from build123d import *

# Parameters (mm, degrees)
SM_BASE_FLANGE_1_DEPTH = 1.5
OTHER_START            = -10
OTHER_1_DEPTH          = 20
OTHER_1_2_DEPTH        = 20
FILLET_1_R             = 1
SKETCH_7_R             = 1.5
CUT_EXTRUDE_1_DEPTH    = 10
SKETCH_8_R             = 1.5
CUT_EXTRUDE_2_DEPTH    = 10


# Read off the part's stored shape, not the designer's step: 绘制的折弯1
# Sheet-metal steps are written as plain solids
with BuildPart() as part:
    # Sketch 1 → 基体-法兰1 (new body)
    with BuildSketch(Plane.XY):
        Polygon((10, 10), (20, 10), (20, 30), (-20, 30), (-20, 10), (-10, 10), (-10, -10), (10, -10), align=None)
    extrude(amount=-SM_BASE_FLANGE_1_DEPTH)

    # Other 1 outline → Other 1 (cut)
    with BuildSketch(Plane.YZ.offset(OTHER_START)):
        with BuildLine():
            ThreePointArc((10, -1.5), (8.630693606, -1.091650066), (7.708712152, 0))
            Line((7.708712152, 0), (-10, 0))
            Line((-10, 0), (-10, -1.5))
            Line((-10, -1.5), (10, -1.5))
        make_face()
    extrude(amount=OTHER_1_DEPTH, mode=Mode.SUBTRACT)

    # Other 1 2 outline → Other 1 2 (add)
    with BuildSketch(Plane.YZ.offset(OTHER_START)):
        with BuildLine():
            Line((9, 18.251106428), (7.5, 18.251106428))
            Line((7.5, 18.251106428), (7.5, 1))
            ThreePointArc((7.5, 1), (7.552734218, 0.489225891), (7.708712152, 0))
            Line((7.708712152, 0), (10, 0))
            ThreePointArc((10, 0), (9.292893219, 0.292893219), (9, 1))
            Line((9, 1), (9, 18.251106428))
        make_face()
    extrude(amount=OTHER_1_2_DEPTH)

    # 圆角1
    fillet_1_edges = [part.edges().sort_by_distance(p)[0] for p in [
        (10, 8.25, 18.251106428),
        (-10, 8.25, 18.251106428),
        (20, 30, -0.75),
        (-20, 30, -0.75),
        (-20, 10, -0.75),
        (20, 10, -0.75),
    ]]
    fillet(fillet_1_edges, radius=FILLET_1_R)

    # 草图7 → 切除-拉伸1 (cut)
    with BuildSketch(Plane(origin=(0, 0, -1.5), x_dir=(-1, 0, 0), z_dir=(0, 0, -1))):
        with Locations((-13, 25)):
            Circle(SKETCH_7_R)
        with Locations((13, 25)):
            Circle(SKETCH_7_R)
        with Locations((-13, 15)):
            Circle(SKETCH_7_R)
        with Locations((13, 15)):
            Circle(SKETCH_7_R)
    extrude(amount=-CUT_EXTRUDE_1_DEPTH, mode=Mode.SUBTRACT)

    # 草图8 → 切除-拉伸2 (cut)
    with BuildSketch(Plane.XZ.offset(-7.5)):
        with Locations(Location((-5, 13.251106428, 0), (0, 0, 270))):
            Circle(SKETCH_8_R)
        with Locations(Location((5, 13.251106428, 0), (0, 0, 270))):
            Circle(SKETCH_8_R)
        with Locations(Location((-5, 6.251106428, 0), (0, 0, 270))):
            Circle(SKETCH_8_R)
        with Locations(Location((5, 6.251106428, 0), (0, 0, 270))):
            Circle(SKETCH_8_R)
    extrude(amount=-CUT_EXTRUDE_2_DEPTH, mode=Mode.SUBTRACT)


solid = part.part
The listing builds one solid part. Answer for the finished solid, in the listing's coordinates (mm). A direction names the side the tool comes from. Give positions to 0.01 mm unless a question says otherwise; leave off trailing zeros. Write each loop counter-clockwise with the first axis right and the second up, starting at its lowest first coordinate (ties: lowest second). Pieces come first, ordered by that corner, then holes. Notation, with made-up numbers: (83, -28.5) -> (104, -28.5) arc R33 cw to (104, 9.5) -> close; hole circle Ø9 at (82.25, 58.5). An arc over 180 degrees is marked (long way). One line per question, with ' | ' between items. Start each with the question number.
1. Find the intervals of material crossed by probe 1 along Y at (x, z) = (13, -1.05); probe 2 along Z at (x, y) = (7.5, 26); probe 3 along Y at (x, z) = (-5.5, 8.5), in increasing order.
2. Section D-D (x = -7.5) is taken. Determine the outline of the cut face in (y, z).
3. Section B-B (y = 25) is taken. Determine the outline of the cut face in (x, z).
4. Given pin 1 Ø2 at (y, z) = (8, 12) entering from -X; pin 2 Ø0.8 at (x, z) = (-13.5, -1) entering from -Y; pin 3 Ø3 at (x, y) = (9, 18.5) entering from +Z, each flat-ended and moving along its own axis, determine where each tip first touches the part or whether it passes through.
5. Section A-A (x = 5) is taken. Determine the outline of the cut face in (y, z), plus the area to 3 significant figures.
6. Section C-C (z = 6) is taken. Determine the outline of the cut face in (x, y).
7. For a pull along X with two mould halves and no side action, classify faces 4 (the cylindrical face through (5.45, 8.24, 4.82)), 5 (the flat face through (0, 20, -1.5)), 6 (the flat face through (20, 20, -1)) as pulls with the +X half, pulls with the -X half, needs draft (parallel to the pull), parting line crosses it, or undercut.
8. For faces 1 (the flat face through (0, 20, 0)), 2 (the flat face through (-15, 10, -1)), 3 (the flat face through (0, 7.5, 10)), determine the directions among +Z, -Z, +X, -X, +Y, -Y from which every point of the face is accessible in a straight line to the end or side of a thin tool.
Response values:
1) probe 1: 10 to 13.5, 16.5 to 23.5, 26.5 to 30 | probe 2: -1.5 to 0 | probe 3: 7.5 to 9
2) outline: (7.5, 1) arc R2.5 ccw to (10, -1.5) -> (30, -1.5) -> (30, 0) -> (10, 0) arc R1 cw to (9, 1) -> (9, 18.25) -> (7.5, 18.25) -> close
3) outline: (-20, -1.5) -> (-14.5, -1.5) -> (-14.5, 0) -> (-20, 0) -> close; (-11.5, -1.5) -> (11.5, -1.5) -> (11.5, 0) -> (-11.5, 0) -> close; (14.5, -1.5) -> (20, -1.5) -> (20, 0) -> (14.5, 0) -> close
4) pin 1: x = -10 | pin 2: y = 10 | pin 3: z = 0
5) outline: (7.5, 1) arc R2.5 ccw to (10, -1.5) -> (30, -1.5) -> (30, 0) -> (10, 0) arc R1 cw to (9, 1) -> (9, 4.75) -> (7.5, 4.75) -> close; (7.5, 7.75) -> (9, 7.75) -> (9, 11.75) -> (7.5, 11.75) -> close; (7.5, 14.75) -> (9, 14.75) -> (9, 18.25) -> (7.5, 18.25) -> close | area: 51.0 mm2
6) outline: (-10, 7.5) -> (-6.48, 7.5) -> (-6.48, 9) -> (-10, 9) -> close; (-3.52, 7.5) -> (3.52, 7.5) -> (3.52, 9) -> (-3.52, 9) -> close; (6.48, 7.5) -> (10, 7.5) -> (10, 9) -> (6.48, 9) -> close
7) face 4: undercut | face 5: needs draft | face 6: pulls with the +X half
8) face 1: +Z, +X, -X, +Y | face 2: +Z, -Z, -X, -Y | face 3: +Z, -Z, +X, -X, -Y
